Autodesk Inventor part; units mm, degrees
ref_plane "YZ Plane" through (0, 0, 0) normal (1, 0, 0) x (0, 1, 0)
ref_plane "XZ Plane" through (0, 0, 0) normal (0, 1, 0) x (-1, 0, 0)
ref_plane "XY Plane" through (0, 0, 0) normal (0, 0, 1) x (1, 0, 0)
sketch "Sketch1" plane through (0, 0, 0) normal (0, 1, 0) x (-1, 0, 0)
  line L0 (-50.8, 50.8) -> (768.4516, 50.8)
  line L1 (768.4516, 50.8) -> (768.4516, -352.9076)
  line L2 (768.4516, -352.9076) -> (-50.8, -352.9076)
  line L3 (-50.8, -352.9076) -> (-50.8, 50.8)
  dimension "d48" = 819.2516
  dimension "d49" = 403.7076
extrude "Plate1" add sketch "Sketch1" along normal blind 3.048
sketch "Sketch2" plane through (-768.4516, 0, -349.8596) normal (0, 0, -1) x (-1, 0, 0)
  line L0 (-819.2516, 0) -> (0, 0)
  line L1 (0, 0) -> (0, 25.4)
  line L2 (0, 25.4) -> (-819.2516, 25.4)
  line L3 (-819.2516, 25.4) -> (-819.2516, 0)
edge flange "Flange1" height 25.4 angle 90 thickness 3.048 bend radius 3.048 thickness toward (0, 0, -1) relief tear relief width 3.048 relief depth 1.524 corner gap 3.048 corner form 2 edges at (-358.8258, 3.048, -352.9076) (-768.4516, 3.048, -151.0538) (-358.8258, 3.048, 50.8) (50.8, 3.048, -151.0538) wall of the first edge with corners at (50.8, 0, -349.8596) (-768.4516, 0, -349.8596) (-768.4516, 25.4, -349.8596) (50.8, 25.4, -349.8596)
bend "Bend1"
corner "Corner1"
equation "\"d50\" = BendReliefWidth"
equation "\"d51\" = BendReliefDepth"
equation "\"d52\" = MinimumRemnant"
equation "\"d53\" = BendRadius"
equation "\"d56\" = BendRadius"
equation "\"d57\" = CornerReliefSize"
equation "\"d58\" = GapSize"
equation "\"d59\" = JacobiRadiusSize"
equation "\"BendRadius\" = Thickness"
equation "\"BendReliefWidth\" = Thickness"
equation "\"BendReliefDepth\" = 0.5 * Thickness"
equation "\"CornerReliefSize\" = 4 * Thickness"
equation "\"MinimumRemnant\" = 2 * Thickness"
equation "\"TransitionRadius\" = BendRadius"
equation "\"JacobiRadiusSize\" = BendRadius"
equation "\"GapSize\" = Thickness"
equation "\"d47\" = BendRadius"
properties part number "BellyPan Lexan" material "Polycarbonate, Clear"
Design review of the part built by this model. Coordinates are the model's own, in mm. A direction names the side the tool comes from. Coordinates: 2 decimals unless noted, no trailing zeros. Loops run counter-clockwise (first coordinate to the right, second up) from the corner with the lowest first, then second, coordinate; pieces in that order, holes last.
Item 1: Add section C-C (x = -411). Write out the cut boundary in (y, z), and give its area (3 significant figures).
Completed:
outline: (0, -346.81) arc R6.1 ccw to (6.1, -352.91) - (25.4, -352.91) - (25.4, -349.86) - (6.1, -349.86) arc R3.05 cw to (3.05, -346.81) - (3.05, 44.7) arc R3.05 cw to (6.1, 47.75) - (25.4, 47.75) - (25.4, 50.8) - (6.1, 50.8) arc R6.1 ccw to (0, 44.7) - close
area: 1,350 mm2
Item 2: Add section B-B (z = -256). Write out the cut boundary in (x, y).
Completed:
outline: (-768.45, 6.1) arc R6.1 ccw to (-762.36, 0) - (44.7, 0) arc R6.1 ccw to (50.8, 6.1) - (50.8, 25.4) - (47.75, 25.4) - (47.75, 6.1) arc R3.05 cw to (44.7, 3.05) - (-762.36, 3.05) arc R3.05 cw to (-765.4, 6.1) - (-765.4, 25.4) - (-768.45, 25.4) - close
Item 3: Draft analysis for pull direction Z (two halves, no side actions). For faces 4 (the flat face through (-364, 16, -352.908)), 5 (the flat face through (-364, 16, -349.86)), 6 (the flat face through (47.752, 16, -154)), 7 (the flat face through (-353, 16, 47.752)), state which applies: pulls with the +Z half, pulls with the -Z half, needs draft (parallel to the pull), parting line crosses it, or undercut.
Completed:
face 4: pulls with the -Z half
face 5: undercut
face 6: needs draft
face 7: undercut
Item 4: Clearance check with flat-ended pins moving along their axes: pin 1 (3 mm diameter, centred on y = 2.5, z = -349.5, fed in from -X); pin 2 (1.8 mm diameter, centred on x = 46.5, y = 3.5, fed in from +Z); pin 3 (0.7 mm diameter, centred on x = -763, z = -351, fed in from -Y). State where each tip first meets the part, or that it passes through.
Completed:
pin 1: stops at x = -762.36
pin 2: stops at z = 44.7
pin 3: stops at y = 6.1
Item 5: Wall thickness on L1, parallel to Z at x = -99, y = 12.75; L2, parallel to Z at x = -476.5, y = 5.75; L3, parallel to X at y = 17.5, z = -268.5: over which ranges is each line inside the solid? List them lowest first.
Completed:
L1: z = -352.91 to -349.86, 47.75 to 50.8
L2: z = -352.9 to -349.84, 47.73 to 50.79
L3: x = -768.45 to -765.4, 47.75 to 50.8
Item 6: Add section A-A (y = 12.5). Write out the cut boundary in (x, z), and give its area (3 significant figures).
Completed:
outline: (-768.45, -347.7) - (-765.4, -347.7) - (-765.4, 45.6) - (-768.45, 45.6) - close; (-763.25, -352.91) - (45.6, -352.91) - (45.6, -349.86) - (-763.25, -349.86) - close; (-763.25, 47.75) - (45.6, 47.75) - (45.6, 50.8) - (-763.25, 50.8) - close; (47.75, -347.7) - (50.8, -347.7) - (50.8, 45.6) - (47.75, 45.6) - close
area: 7,330 mm2
Item 7: For faces 1 (the flat face through (-765.404, 16, -148)), 2 (the flat face through (-353, 3.048, -148)), 3 (the flat face through (-353, 0, -148)), list the 3-axis set-ups (+Z, -Z, +X, -X, +Y, -Y) from which the entire face can be reached by the end or side of a thin tool; tool diameter is ignored.
Completed:
face 1: +Z, -Z, +Y
face 2: +Y
face 3: +Z, -Z, +X, -X, -Y
